Autodesk Inventor part; units mm, degrees
ref_plane "YZ Plane" through (0, 0, 0) normal (1, 0, 0) x (0, 1, 0)
ref_plane "XZ Plane" through (0, 0, 0) normal (0, 1, 0) x (-1, 0, 0)
ref_plane "XY Plane" through (0, 0, 0) normal (0, 0, 1) x (1, 0, 0)
sketch "Sketch1" plane through (0, 0, 0) normal (0, 1, 0) x (-1, 0, 0)
  line L0 (10.6592, 57.15) -> (-7.8828, 57.15)
  line L1 (-7.8828, 57.15) -> (-7.8828, -12.7)
  line L2 (-7.8828, -12.7) -> (10.6592, -12.7)
  line L3 (10.6592, 51.435) -> (-1.5328, 51.435)
  line L4 (-1.5328, 51.435) -> (-1.5328, 25.4)
  line L5 (-1.5328, 25.4) -> (10.6592, 25.4)
  line L6 (10.6592, 19.05) -> (-1.5328, 19.05)
  line L7 (-1.5328, 19.05) -> (-1.5328, -6.35)
  line L8 (-1.5328, -6.35) -> (10.6592, -6.35)
  line L9 (10.6592, -12.7) -> (10.6592, -6.35)
  line L10 (10.6592, 19.05) -> (10.6592, 25.4)
  line L11 (10.6592, 51.435) -> (10.6592, 57.15)
  point P0 (0, 0)
  dimension "d0" = 18.542
  dimension "d3" = 6.35
  dimension "d4" = 6.35
  dimension "d5" = 5.715
  dimension "d7" = 0
  dimension "d8" = 26.035
  dimension "d9" = 25.4
  dimension "d25" = 0
  dimension "d26" = 0
extrude "Extrusion1" add sketch "Sketch1" along normal blind 101.6
sketch "Sketch2" plane through (1.5328, 0, -6.35) normal (-1, 0, 0) x (0, 0, 1)
  line L0 (0, 0) -> (0, 101.6)
  line L1 (0, 0) -> (25.4, 0)
  point P0 (6.35, 0)
  point P1 (12.7, 25.4)
  point P2 (12.7, 50.8)
  point P3 (12.7, 76.2)
  dimension "d12" = 12.7
  dimension "d13" = 25.4
  dimension "d14" = 25.4
  dimension "d15" = 0
  dimension "d16" = 0
  dimension "d17" = 25.4
hole "Hole1" at (1.5328, 25.4, 6.35) at (1.5328, 50.8, 6.35) at (1.5328, 76.2, 6.35) direction (1, 0, 0) diameter 4.826 depth 25.4 tip angle 118
sketch "Sketch3" plane through (0, 101.6, 0) normal (0, 1, 0) x (1, 0, 0)
  line L0 (1.5328, -25.4) -> (-10.7917, -24.9696)
  line L1 (-10.7917, -24.9696) -> (-10.7917, -25.4)
  line L2 (-10.6592, -25.4) -> (1.5328, -25.4)
  line L3 (-10.7917, -25.4) -> (1.5328, -25.4)
  point P0 (0, 0)
  dimension "d27" = 2
extrude "Extrusion2" cut sketch "Sketch3" against normal blind 111.125
sketch "Sketch4" plane through (0, 101.6, 0) normal (0, 1, 0) x (1, 0, 0)
  line L0 (1.5328, -51.435) -> (-12.9577, -51.435)
  line L1 (-12.9577, -51.435) -> (-12.9577, -51.941)
  line L2 (-12.9577, -51.941) -> (1.5328, -51.435)
  point P0 (0, 0)
  dimension "d30" = 2
extrude "Extrusion3" cut sketch "Sketch4" against normal blind 119.0625
sketch "Sketch5" plane through (0, 101.6, 0) normal (0, 1, 0) x (1, 0, 0)
  line L0 (-10.6592, -57.15) -> (7.8828, -57.15)
  line L1 (7.8828, -57.15) -> (-13.0423, -56.4193)
  line L2 (-13.0423, -56.4193) -> (-13.0009, -57.15)
  line L3 (-13.0009, -57.15) -> (7.8828, -57.15)
  point P0 (0, 0)
  dimension "d33" = 2
extrude "Extrusion4" cut sketch "Sketch5" against normal blind 196.85
sketch "Sketch6" plane through (0, 101.6, 0) normal (0, 1, 0) x (1, 0, 0)
  line L0 (7.8828, 12.7) -> (-10.6592, 12.7)
  line L1 (7.8828, 12.7) -> (-16.8119, 12.7)
  line L2 (-16.8119, 12.7) -> (-16.8119, 11.8376)
  line L3 (7.8828, -57.15) -> (7.8828, 12.7)
  line L4 (-16.8119, 11.8376) -> (7.8828, 12.7)
  point P0 (0, 0)
  dimension "d36" = 2
extrude "Extrusion5" cut sketch "Sketch6" against normal blind 334.9625
sketch "Sketch8" plane through (1.5328, 0, -6.35) normal (-1, 0, 0) x (0, 0, 1)
  line L0 (0, 0) -> (25.4, 0)
  circle A0 centre (12.7, 25.4) radius 2.413
  circle A1 centre (12.7, 50.8) radius 2.413
  circle A2 centre (12.7, 76.2) radius 2.413
  line L1 (25.4, 0) -> (25.4, 101.6)
  line L2 (0, 0) -> (25.4, 0)
  line L3 (25.4, 0) -> (25.4, 101.6)
  line L4 (25.4, 101.6) -> (0, 101.6)
  line L5 (0, 101.6) -> (0, 0)
  circle A3 centre (12.7, 25.4) radius 2.413
  circle A4 centre (12.7, 50.8) radius 2.413
  circle A5 centre (12.7, 76.2) radius 2.413
  point P0 (6.35, 0)
extrude "Extrusion7" add sketch "Sketch8" along normal blind 1.1906
sketch "Sketch9" plane through (1.5328, 0, 25.4) normal (-1, 0, 0) x (0, 0, 1)
  line L0 (10.16, 48.26) -> (15.24, 48.26)
  line L1 (15.24, 48.26) -> (15.24, 53.34)
  line L2 (15.24, 53.34) -> (10.16, 53.34)
  line L3 (10.16, 53.34) -> (10.16, 48.26)
  line L4 (0, 101.6) -> (26.035, 101.6)
  line L5 (0, 0) -> (0, 101.6)
  point P0 (-25.4, 0)
  dimension "d43" = 5.08
  dimension "d44" = 5.08
  dimension "d45" = 48.26
  dimension "d46" = 10.16
extrude "Extrusion8" cut sketch "Sketch9" against normal blind 19.4469
equation "\"d0\" = ElvDelWidth"
equation "\"d3\" = ElvDelFrontTabLength"
equation "\"d4\" = ElvDelMiddleTabLength"
equation "\"d9\" = ElvBeamWidth"
equation "\"d10\" = ElvDelHeight"
equation "\"ElvBeamWidth\" = 25.4"
equation "\"ElvDelWidth\" = 18.542"
equation "\"ElvDelHeight\" = 101.6"
equation "\"ElvDelFrontTabLength\" = 6.35"
equation "\"ElvDelDepth\" = 6.35"
equation "\"d2\" = ElvDelDepth"
equation "\"ElvCrossBeamLength\" = 304.8"
equation "\"ElvFixedBeamLength\" = 990.6"
equation "\"ElvMiddleBeamLength\" = 990.6"
equation "\"ElvFrontBeamLength\" = 990.6"
equation "\"ElvEndEffectLength\" = 431.8"
equation "\"ElvWallWidth\" = 1.5875"
equation "\"ElvTopBeamLength\" = 457.2"
equation "\"ElvHoleFromFront\" = 25.4"
equation "\"ElvHoleFromMid\" = 38.1"
equation "\"ElvHoleFromFixed\" = 50.8"
equation "\"ElvHoleFromBottom\" = 38.1"
equation "\"ElvRivetPlateLength\" = 76.2"
equation "\"ElvDelMiddleTabLength\" = 6.35"
properties part number "ElvDelV4" material "Acetal Resin, White"
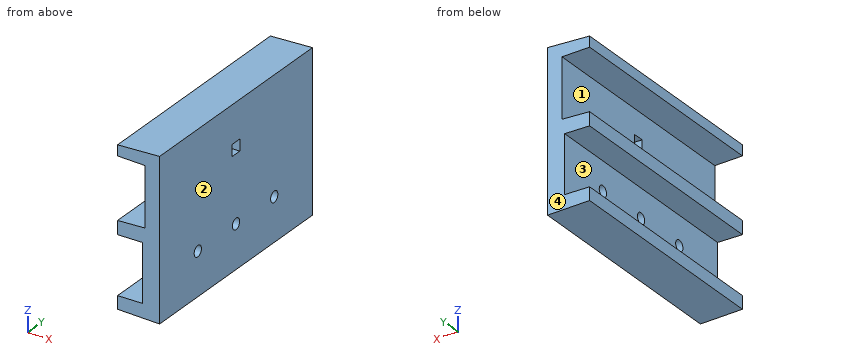
Geometry check sheet. Reference: the model listing, model coordinates, mm. Face numbers are marked on the shaded views. A direction names the side the tool comes from. Round coordinates to 2 decimals unless told otherwise and drop trailing zeros. Order: outer loops, then holes, each group sorted by start corner. A loop starts at its lowest first (then second) coordinate and runs counter-clockwise, first axis right, second up. Notation, with made-up numbers: (42.5, 54.25) - (99.5, 54.25) arc R30 ccw to (99.5, 76.25) - close; hole circle Ø9 at (38, 75.25). An arc over 180 degrees is marked (long way). One line per question, with ' | ' between items. Start each with the question number.
(1) Sectioned sample at D-D on x = 4. Record the cut outline in (y, z), and give its area (3 significant figures).
(2) Sectioned sample at C-C on z = 6.35. Record the cut outline in (x, y), and give its area (3 significant figures).
(3) Thickness scan on L1, parallel to Y at x = 3.5, z = 6.35; L2, parallel to Z at x = -3.25, y = 41.5; L3, parallel to Y at x = 1.75, z = 7.5. Record the ranges inside material, lowest first. Write a range as [from, to].
(4) Access from +Z, -Z, +X, -X, +Y, -Y to the whole of each face (thin tool, end or side, straight path). Record for the marked faces 1 and 2.
(5) Release check for a two-part mould opening along Z. For the marked faces 3 and 4 record: released by +Z, released by -Z, zero draft, split by the parting line, or undercut.
(6) Sectioned sample at A-A on y = 50.8. Record the cut outline in (x, z) (3 decimals).
(7) Sectioned sample at B-B on y = 76.2. Record the cut outline in (x, z) (3 decimals), and give its area (3 significant figures).
(8) Depth check by flat-ended pin: pin 1 Ø8 at (x, y) = (-4, 29.5) entering from -Z; pin 2 Ø5.5 at (x, y) = (5.5, 51.5) entering from -Z; pin 3 Ø4.5 at (y, z) = (76.2, 6.35) entering from +X; pin 4 Ø3.5 at (x, y) = (-6.5, 73) entering from -Z. Enter the tip coordinate at first touch or a pass-through.
Conclusion:
1) outline: (0, -12.56) - (101.6, -12.56) - (101.6, 57.01) - (0, 57.01) - close; hole circle Ø4.83 at (25.4, 6.35); hole (48.26, 35.56) - (53.34, 35.56) - (53.34, 40.64) - (48.26, 40.64) - close; hole circle Ø4.83 at (50.8, 6.35); hole circle Ø4.83 at (76.2, 6.35) | area: 6,990 mm2
2) outline: (0.34, 0) - (7.88, 0) - (7.88, 22.99) - (0.34, 22.99) - close; (0.34, 27.81) - (7.88, 27.81) - (7.88, 48.39) - (0.34, 48.39) - close; (0.34, 53.21) - (7.88, 53.21) - (7.88, 73.79) - (0.34, 73.79) - close; (0.34, 78.61) - (7.88, 78.61) - (7.88, 101.6) - (0.34, 101.6) - close | area: 657 mm2
3) L1: y = [0, 22.99], [27.81, 48.39], [53.21, 73.79], [78.61, 101.6] | L2: z = [-12.31, -6.35], [19.05, 25.23], [51.6, 56.76] | L3: y = [0, 23.28], [27.52, 48.68], [52.92, 74.08], [78.32, 101.6]
4) face 1: -X, +Y, -Y | face 2: +Z, -Z, +X, +Y, -Y
5) face 3: undercut | face 4: zero draft
6) outline: (-10.659, -12.052) - (7.883, -12.7) - (7.883, 3.937) - (0.342, 3.937) - (0.342, -6.35) - (-10.659, -6.35) - close; (-10.659, 19.05) - (0.342, 19.05) - (0.342, 8.763) - (7.883, 8.763) - (7.883, 35.56) - (1.533, 35.56) - (1.533, 25.4) - (-10.659, 24.974) - close; (-10.659, 51.861) - (1.533, 51.435) - (1.533, 40.64) - (7.883, 40.64) - (7.883, 57.15) - (-10.659, 56.503) - close
7) outline: (-10.659, -12.052) - (7.883, -12.7) - (7.883, 3.937) - (0.342, 3.937) - (0.342, -6.35) - (-10.659, -6.35) - close; (-10.659, 19.05) - (0.342, 19.05) - (0.342, 8.763) - (7.883, 8.763) - (7.883, 57.15) - (-10.659, 56.503) - (-10.659, 51.861) - (1.533, 51.435) - (1.533, 25.4) - (-10.659, 24.974) - close | area: 645 mm2
8) pin 1: stops at z = -12.42 | pin 2: stops at z = -12.7 | pin 3: passes through | pin 4: stops at z = -12.26
